from build123d import *

# Parameters (mm, degrees)
SKETCH1_R           = 4
SKETCH1_R_2         = 1.5
BOSS_EXTRUDE1_DEPTH = 2
SKETCH2_R           = 4
SKETCH2_R_2         = 1.5
BOSS_EXTRUDE2_DEPTH = 2
FILLET1_R           = 1
FILLET3_R           = 2


with BuildPart() as part:
    # Sketch1 → Boss-Extrude1 (new body)
    with BuildSketch(Plane(origin=(0, 0, 0), x_dir=(1, 0, 0), z_dir=(0, 1, 0))):
        with BuildLine():
            Line((0, 12.5), (0, -12.5))
            Line((0, -12.5), (-19.5, -12.5))
            ThreePointArc((-19.5, -12.5), (-32, 0), (-19.5, 12.5))
            Line((-19.5, 12.5), (0, 12.5))
        make_face()
        with Locations(Location((-19.5, 0, 0), (0, 0, 270))):
            Circle(SKETCH1_R, mode=Mode.SUBTRACT)
        with Locations(Location((-19.5, 7, 0), (0, 0, 270))):
            Circle(SKETCH1_R_2, mode=Mode.SUBTRACT)
        with Locations(Location((-19.5, -7, 0), (0, 0, 270))):
            Circle(SKETCH1_R_2, mode=Mode.SUBTRACT)
        with Locations(Location((-12.5, 0, 0), (0, 0, 270))):
            Circle(SKETCH1_R_2, mode=Mode.SUBTRACT)
        with Locations(Location((-26.5, 0, 0), (0, 0, 270))):
            Circle(SKETCH1_R_2, mode=Mode.SUBTRACT)
    extrude(amount=BOSS_EXTRUDE1_DEPTH)

    # Sketch2 → Boss-Extrude2 (add)
    with BuildSketch(Plane(origin=(0, 0, 0), x_dir=(0, 0, -1), z_dir=(1, 0, 0))):
        with BuildLine():
            Line((-12.5, 0), (12.5, 0))
            Line((12.5, 0), (12.5, 14))
            ThreePointArc((12.5, 14), (0, 26.5), (-12.5, 14))
            Line((-12.5, 14), (-12.5, 0))
        make_face()
        with Locations((0, 14)):
            Circle(SKETCH2_R, mode=Mode.SUBTRACT)
        with Locations((0, 21)):
            Circle(SKETCH2_R_2, mode=Mode.SUBTRACT)
        with Locations((7, 14)):
            Circle(SKETCH2_R_2, mode=Mode.SUBTRACT)
        with Locations((0, 7)):
            Circle(SKETCH2_R_2, mode=Mode.SUBTRACT)
        with Locations((-7, 14)):
            Circle(SKETCH2_R_2, mode=Mode.SUBTRACT)
    extrude(amount=BOSS_EXTRUDE2_DEPTH)

    # Fillet1
    fillet1_edges = [part.edges().sort_by_distance(p)[0] for p in [
        (0, 2, 0),
    ]]
    fillet(fillet1_edges, radius=FILLET1_R)

    # Fillet3
    fillet3_edges = [part.edges().sort_by_distance(p)[0] for p in [
        (2, 0, 0),
    ]]
    fillet(fillet3_edges, radius=FILLET3_R)


solid = part.part
Model file for the job. Use its own axes, mm. A direction names the side the tool comes from. Coordinates: 2 decimals unless noted, no trailing zeros. Loops run counter-clockwise (first coordinate to the right, second up) from the corner with the lowest first, then second, coordinate; pieces in that order, holes last. Notation, with made-up numbers: (23.5, -38) -> (71.5, -38) arc R30 cw to (71.5, -7) -> close; hole circle Ø5 at (-27, 72.25). An arc over 180 degrees is marked (long way). Use one line per item in the form item = value. Start each with the question number.
(1) Cut at C-C on z = -7. Give the cut face in (x, y), and give its area (3 significant figures).
(2) Probe probe 1 along X at (y, z) = (1.4, 0); probe 2 along Y at (x, z) = (0.7, 0); probe 3 along X at (y, z) = (12.75, 8). List the from-to ranges inside material, lowest first. Write a range as from..to.
(3) Tool access for faces 1 (the cylindrical face through (0.986, 5.536, 0.325)), 2 (the flat face through (-16, 2, -3)): list every direction of +Z, -Z, +X, -X, +Y, -Y with a clear straight run to the whole face (end or side of a thin tool).
(4) Cut at B-B on y = 7. Give the cut face in (x, z).
(5) Cut at D-D on y = 21. Give the cut face in (x, z).
(6) Flat gauge pins, fed straight in: pin 1 (1 mm diameter, centred on x = -19.5, z = 4, fed in from -Y); pin 2 (7.5 mm diameter, centred on x = -15, z = -3.5, fed in from +Y); pin 3 (3.5 mm diameter, centred on y = 14, z = 7, fed in from -X). Where does each tip first touch, or does it go through?
(7) Pull direction X, two halves, no side cores. Call faces 3 (the cylindrical face through (0.99, 14.07, -5.5)), 4 (the cylindrical face through (-18.49, 0.99, -8.11)), 5 (the flat face through (0, 9.7, 0.2)): pulls with the +X half, pulls with the -X half, needs draft (parallel to the pull), parting line crosses it, or undercut.
(8) Cut at A-A on z = 0. Give the number of separate pieces and of enclosed holes in the cut face, and give its area (3 significant figures).
Values:
q1.outline = (-29.86, 0) -> (-21, 0) -> (-21, 2) -> (-29.86, 2) -> close; (-18, 0) -> (0, 0) arc R2 ccw to (2, 2) -> (2, 12.5) -> (0, 12.5) -> (0, 3) arc R1 cw to (-1, 2) -> (-18, 2) -> close; (0, 15.5) -> (2, 15.5) -> (2, 24.36) -> (0, 24.36) -> close
q1.area = 95.8 mm2
q2.probe_1 = -32..-28, -25..-23.5, -15.5..-14, -11..1.91
q2.probe_2 = 0.13..5.5, 8.5..10, 18..19.5, 22.5..26.5
q2.probe_3 = 0..2
q3.face_1 = +X, -X
q3.face_2 = +Z, -Z, -X, +Y
q4.outline = (0, -12.5) -> (2, -12.5) -> (2, -1.5) -> (0, -1.5) -> close; (0, 1.5) -> (2, 1.5) -> (2, 12.5) -> (0, 12.5) -> close
q5.outline = (0, -10.36) -> (2, -10.36) -> (2, -1.5) -> (0, -1.5) -> close; (0, 1.5) -> (2, 1.5) -> (2, 10.36) -> (0, 10.36) -> close
q6.pin_1 = 0
q6.pin_2 = 2
q6.pin_3 = 0
q7.face_3 = needs draft
q7.face_4 = undercut
q7.face_5 = pulls with the -X half
q8.separate_pieces = 7
q8.enclosed_holes = 0
q8.area = 60.4 mm2
